Here's how the part is built. I have some questions about the finished solid (model axes, mm). Coordinates: 2 decimals unless noted, no trailing zeros. Loops run counter-clockwise (first coordinate to the right, second up) from the corner with the lowest first, then second, coordinate; pieces in that order, holes last.
```python
from build123d import *

# Parameters (mm, degrees)
F0_W     = 381
F0_H     = 381
F0_W_2   = 19.05
F0_H_2   = 101.6
F1_DEPTH = 19.05


with BuildPart() as f1:
    # F0 (on Top) → F1 (new body)
    with BuildSketch(Plane.XY):
        with Locations((431.801737, 1589.52043)):
            Rectangle(F0_W, F0_H)
        Polygon((47.983605, 364.294128), (46.651042, -124.97957), (808.651042, -124.97957), (812.801737, 1399.02043), (622.301737, 1399.02043), (241.301737, 1399.02043), (50.818977, 1399.02043), (50.818977, 1405.350483), align=None)
        Polygon((148.593587, 0.653433), (149.583228, 364.017416), (150.115503, 559.451361), (251.715126, 559.174649), (250.19321, 0.376722), align=None, mode=Mode.SUBTRACT)
        with Locations((298.59611, 564.617765)):
            Rectangle(F0_W_2, F0_H_2, mode=Mode.SUBTRACT)
        Polygon((355.601737, 558.717186), (431.801737, 558.381641), (508.001737, 558.037416), (508.001737, -0.759322), (429.341096, -0.412941), (353.139618, -0.412941), align=None, mode=Mode.SUBTRACT)
        Polygon((548.521661, 512.759166), (549.416431, 614.355226), (568.465692, 614.187457), (567.570922, 512.591397), align=None, mode=Mode.SUBTRACT)
    extrude(amount=F1_DEPTH)


solid = f1.part
```
1. I want a section at A-A (z = 15.25). Please give me the cut outline in (x, y), then the cut area to 3 significant figures.
2. I want a section at D-D (y = 235.5). Please give me the cut outline in (x, z).
3. I want a section at C-C (x = 491). Please give me the cut outline in (y, z), then the cut area to 3 significant figures.
4. I want a section at B-B (y = 537). Please give me the cut outline in (x, z).
5. For pin 1 (1 mm diameter, centred on y = 1286.5, z = 9.5, fed in from -X); pin 2 (10 mm diameter, centred on y = 194, z = 5, fed in from +X); pin 3 (2 mm diameter, centred on y = 792, z = 9.5, fed in from +X), each with a flat end and sliding along its axis, tell me the tip position at first contact or that it passes through.
6. I need wall thicknesses on line 1 along Y through (x, z) = (212, 17.5); line 2 along Y through (x, z) = (484, 11.5); line 3 along X through (y, z) = (1266, 1). Which ranges of each line are inside material? Lowest first, please.
Response values:
1. outline: (46.65, -124.98) - (808.65, -124.98) - (812.8, 1399.02) - (622.3, 1399.02) - (622.3, 1780.02) - (241.3, 1780.02) - (241.3, 1399.02) - (50.82, 1399.02) - (50.82, 1405.35) - close; hole (148.59, 0.65) - (250.19, 0.38) - (251.72, 559.17) - (150.12, 559.45) - close; hole (289.07, 513.82) - (308.12, 513.82) - (308.12, 615.42) - (289.07, 615.42) - close; hole (353.14, -0.41) - (429.34, -0.41) - (508, -0.76) - (508, 558.04) - (431.8, 558.38) - (355.6, 558.72) - close; hole (548.52, 512.76) - (567.57, 512.59) - (568.47, 614.19) - (549.42, 614.36) - close
1. area: 1,160,000 mm2
2. outline: (47.63, 0) - (149.23, 0) - (149.23, 19.05) - (47.63, 19.05) - close; (250.83, 0) - (354.18, 0) - (354.18, 19.05) - (250.83, 19.05) - close; (508, 0) - (809.63, 0) - (809.63, 19.05) - (508, 19.05) - close
3. outline: (-124.98, 0) - (-0.68, 0) - (-0.68, 19.05) - (-124.98, 19.05) - close; (558.11, 0) - (1780.02, 0) - (1780.02, 19.05) - (558.11, 19.05) - close
3. area: 25,600 mm2
4. outline: (48.45, 0) - (150.05, 0) - (150.05, 19.05) - (48.45, 19.05) - close; (251.65, 0) - (289.07, 0) - (289.07, 19.05) - (251.65, 19.05) - close; (308.12, 0) - (355.51, 0) - (355.51, 19.05) - (308.12, 19.05) - close; (508, 0) - (548.74, 0) - (548.74, 19.05) - (508, 19.05) - close; (567.79, 0) - (810.45, 0) - (810.45, 19.05) - (567.79, 19.05) - close
5. pin 1: stops at x = 50.49
5. pin 2: stops at x = 809.53
5. pin 3: stops at x = 811.15
6. line 1: y = -124.98 to 0.48, 559.28 to 1399.02
6. line 2: y = -124.98 to -0.65, 558.15 to 1780.02
6. line 3: x = 50.44 to 812.44
